```python
from build123d import *

# Parameters (mm, degrees)
F0_W      = 50
F0_H      = 50
F1_DEPTH  = 500
F3_W      = 50
F3_H      = 50
F4_ANGLE  = 90
F5_ANGLE  = 90
F4_FACE_W = 50
F4_FACE_H = 50
F5_FACE_W = 50
F5_FACE_H = 50
F7_DEPTH  = 500
F8_W      = 50
F8_H      = 50
F9_ANGLE  = 90
F10_DEPTH = 1500


with BuildPart() as f1:
    # F0 (on Front) → F1 (new body, symmetric)
    with BuildSketch(Plane.XZ):
        with Locations((475, 25)):
            Rectangle(F0_W, F0_H)
    extrude(amount=F1_DEPTH, both=True)

    # F3 (on offset) → F5 (revolve)
    with BuildSketch(Plane.XZ.offset(500)):
        with Locations((475, 25)):
            Rectangle(F3_W, F3_H)
    revolve(axis=Axis((350, -500, -3.7102438509), (0, 0, -1)), revolution_arc=F5_ANGLE)



with BuildPart() as f1b:
    # F0 (on Front) → F1, piece 2 (new body, symmetric)
    with BuildSketch(Plane.XZ):
        with Locations((-475, -25)):
            Rectangle(F0_W, F0_H)
    extrude(amount=F1_DEPTH, both=True)

    # F3 (on offset) → F4 (revolve)
    with BuildSketch(Plane.XZ.offset(500)):
        with Locations((-475, -25)):
            Rectangle(F3_W, F3_H)
    revolve(axis=Axis((-350, -500, -32.6501708478), (0, 0, 1)), revolution_arc=F4_ANGLE)


with BuildPart() as f1_1:
    add(f1.part)

    add(f1b.part)  # F6 merges F1b
    # F4_face (on face) → F6 section 0
    with BuildSketch(Plane(origin=(-350, -625, -25), x_dir=(0, 1, 0), z_dir=(1, 0, 0))):
        Rectangle(F4_FACE_W, F4_FACE_H)
    # F5_face (on face) → F6 section 1
    with BuildSketch(Plane(origin=(350, -625, 25), x_dir=(0, -1, 0), z_dir=(-1, 0, 0))):
        Rectangle(F5_FACE_W, F5_FACE_H)
    loft()

    # F7 (add): a face of the model
    f7_faces = [f1_1.faces().sort_by_distance(p)[0] for p in [
        (-475, 500, -25),
    ]]
    extrude(f7_faces, amount=F7_DEPTH)

    # F8 (on face) → F9 (revolve)
    with BuildSketch(Plane(origin=(0, 500, 0), x_dir=(-1, 0, 0), z_dir=(0, 1, 0))):
        with Locations((-475, 25)):
            Rectangle(F8_W, F8_H)
    revolve(axis=Axis((350, 500, -1.4840960503), (0, 0, 1)), revolution_arc=F9_ANGLE)

    # F10 (add): a face of the model
    f10_faces = [f1_1.faces().sort_by_distance(p)[0] for p in [
        (350, 625, 25),
    ]]
    extrude(f10_faces, amount=F10_DEPTH)


solid = f1_1.part
```
Build history of the part. All positions in model axes, mm. A direction names the side the tool comes from. Give positions to 0.01 mm unless a question says otherwise; leave off trailing zeros. Order: outer loops, then holes, each group sorted by start corner. A loop starts at its lowest first (then second) coordinate and runs counter-clockwise, first axis right, second up. Notation, with made-up numbers: M 9.25,21 L 22.25,21 A28 cw 22.25,57 Z; hole C -4.75,54 d6. An arc over 180 degrees is marked long. Write item = value, one per line. Start each with the question number.
(1) Slice it at C-C on x = -530. Write the cut outline in (y, z), plus the area to 3 significant figures.
(2) Two-plate mould, pull along Y, no slides. Class faces 6 (the cylindrical face through (-457.23, -604.89, -24.65)), 7 (the flat face through (485, 292, 0)), 8 (the cylindrical face through (421.484, 569.929, 25.35)), 9 (the flat face through (-389, 600, 25)): released by +Y, released by -Y, zero draft, split by the parting line, or undercut.
(3) Which spindle directions (+Z, -Z, +X, -X, +Y, -Y) get a long thin tool onto all of the face, cutting with end or side? Do faces 1 (the flat face through (4.9, -624.65, 25.35)), 2 (the flat face through (-475, 823, 0)), 3 (the cylindrical face through (421.484, -569.929, 25.35)), 4 (the flat face through (4.9, -625.35, -24.65)), 5 (the cylindrical face through (-421.484, -569.929, -24.65)). Say none if no direction does.
(4) Slice it at B-B on x = 376. Write the cut outline in (y, z), plus the area to 3 significant figures.
(5) Pin check, flat tips, straight feed: pin 1 Ø15 at (x, z) = (-283.5, 32.5) entering from -Y; pin 2 Ø25 at (x, y) = (-689, 635.5) entering from -Z; pin 3 Ø12 at (x, z) = (51.5, -17.5) entering from +Y. Stop position of each tip, or through.
(6) Slice it at A-A on y = 15. Write the cut outline in (x, z).
(7) Probe L1, parallel to Y at x = 269, z = 14; L2, parallel to X at y = 40, z = 39.5; L3, parallel to Y at x = -395, z = 0.5. List the from-to ranges inside material, lowest first. Write a range as [from, to].
Responses:
q1.outline = M 600,0 L 650,0 L 650,50 L 600,50 Z
q1.area = 2,500 mm2
q2.face_6 = released by -Y
q2.face_7 = zero draft
q2.face_8 = undercut
q2.face_9 = undercut
q3.face_1 = +Z, -X, -Y
q3.face_2 = +Z, +X, -X, +Y
q3.face_3 = +Z, -Z, -X
q3.face_4 = -Z, +X, +Y, -Y
q3.face_5 = +Z, -Z, +X, +Y
q4.outline = M -647.73,0 L -596.56,0 L -596.56,50 L -647.73,50 Z; M 596.56,0 L 647.73,0 L 647.73,50 L 596.56,50 Z
q4.area = 5,120 mm2
q5.pin_1 = 600
q5.pin_2 = 0
q5.pin_3 = -600
q6.outline = M -500,-50 L -450,-50 L -450,0 L -500,0 Z; M 450,0 L 500,0 L 500,50 L 450,50 Z
q7.L1 = [-650, -600], [600, 650]
q7.L2 = [450, 500]
q7.L3 = [600, 650]
